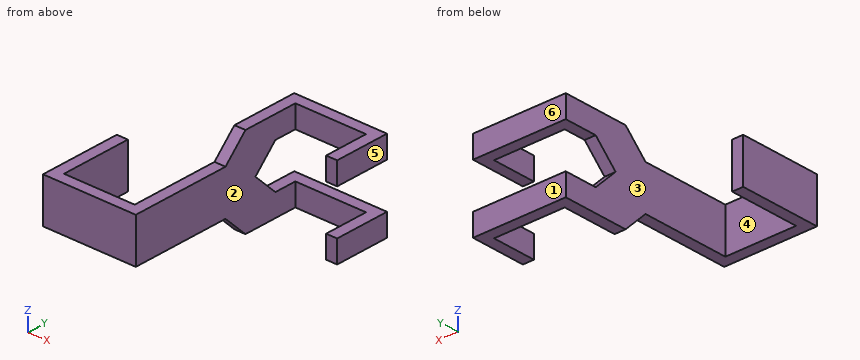
from build123d import *

# Parameters (mm, degrees)
F1_DEPTH = 5
F2_W     = 2.5
F2_H     = 2.5
F3_DEPTH = 5
F5_DEPTH = 2.5


with BuildPart() as f1:
    # F0 (on Top) → F1 (new body)
    with BuildSketch(Plane.XY):
        Polygon((-16, -30), (-16, 0), (-18.5, 0), (-18.5, -27.5), (-34.5, -27.5), (-34.5, -11.5), (-37, -11.5), (-37, -30), align=None)
    extrude(amount=F1_DEPTH)

    # F2 (on face) → F3 (join)
    with BuildSketch(Plane.XY.offset(5)):
        Polygon((2.5, 12.5), (-18.5, 12.5), (-18.5, 0), (-16, 0), (-16, 10), (0, 10), (0, 0), (2.5, 0), align=None)
        with Locations((-17.25, -1.25)):
            Rectangle(F2_W, F2_H)
    extrude(amount=F3_DEPTH)

    # F4 (on face) → F5 (join, through all)
    with BuildSketch(Plane(origin=(-18.5, 0, 0), x_dir=(0, -1, 0), z_dir=(-1, 0, 0))):
        Polygon((0, 5), (-5, 5), (0, 0), align=None)
        Polygon((7.5, 5), (2.5, 10), (2.5, 5), align=None)
    extrude(amount=-F5_DEPTH)

    # F6: F1 across plane


with BuildPart() as f1_1:
    add(f1.part)
    add(f1.part.mirror(Plane.XY))


solid = f1_1.part
Source: CAD feature listing. Evaluate the final solid. Frame: model axes, mm. Face numbers are marked on the shaded views. A direction names the side the tool comes from. Coordinates: 2 decimals unless noted, no trailing zeros. Loops run counter-clockwise (first coordinate to the right, second up) from the corner with the lowest first, then second, coordinate; pieces in that order, holes last. Notation, with made-up numbers: (75, 22.5) -> (122, 22.5) arc R15 ccw to (122, 33.5) -> close; hole circle Ø4 at (47, 76). An arc over 180 degrees is marked (long way). Answer in a Markdown table with one row per item. Add a question column.
Q1. Reachability of the marked faces 1, 2 and 3 from +Z, -Z, +X, -X, +Y, -Y: full face, straight path, thin tool, end or side. Return the list, or none.
Q2. Contact query for flat-ended pins moving along their axis: pin 1 Ø2.5 at (x, z) = (-10.5, 6.5) entering from -Y; pin 2 Ø3 at (x, z) = (2, -7) entering from -Y; pin 3 Ø5.5 at (y, z) = (5.5, -8) entering from -X. Output: stop coordinate, or through.
Q3. Section A-A on y = 0.5. Return the cut outline in (x, z).
Q4. Pull-direction query (X, two-part tool) for the marked faces 4, 5 and 6; classes: pulls with the +X half, pulls with the -X half, needs draft (parallel to the pull), parting line crosses it, or undercut.
Q5. Section D-D on y = -16. Return the cut outline in (x, z), and give its area (3 significant figures).
Q6. Section B-B on x = -2. Return the cut outline in (y, z).
Q7. Section C-C on z = 3.5. Return the cut outline in (x, y).
Q8. Ray query, line 1 along Z through (x, y) = (-14.5, 11); line 2 along X through (y, z) = (-22, 4.5); line 3 along X through (y, z) = (1.5, -8.25). Return the intervals inside material, ascending.
Computed values:
| question | item | result |
|---|---|---|
| 1 | face 1 | +Z, -Z, +X, -X, +Y |
| 1 | face 2 | +Z, -Z, -Y |
| 1 | face 3 | +Z, -Z, +Y |
| 2 | pin 1 | stops at y = 10 |
| 2 | pin 2 | stops at y = 0 |
| 2 | pin 3 | stops at x = -18.5 |
| 3 | outline | (-18.5, -10) -> (-16, -10) -> (-16, -0.5) -> (-18.5, -0.5) -> close; (-18.5, 0.5) -> (-16, 0.5) -> (-16, 10) -> (-18.5, 10) -> close; (0, -10) -> (2.5, -10) -> (2.5, -5) -> (0, -5) -> close; (0, 5) -> (2.5, 5) -> (2.5, 10) -> (0, 10) -> close |
| 4 | face 4 | undercut |
| 4 | face 5 | pulls with the +X half |
| 4 | face 6 | needs draft |
| 5 | outline | (-37, -5) -> (-34.5, -5) -> (-34.5, 5) -> (-37, 5) -> close; (-18.5, -5) -> (-16, -5) -> (-16, 5) -> (-18.5, 5) -> close |
| 5 | area | 50.0 mm^2 |
| 6 | outline | (10, -10) -> (12.5, -10) -> (12.5, -5) -> (10, -5) -> close; (10, 5) -> (12.5, 5) -> (12.5, 10) -> (10, 10) -> close |
| 7 | outline | (-37, -30) -> (-16, -30) -> (-16, 3.5) -> (-18.5, 3.5) -> (-18.5, -27.5) -> (-34.5, -27.5) -> (-34.5, -11.5) -> (-37, -11.5) -> close |
| 8 | line 1 | z = -10 to -5, 5 to 10 |
| 8 | line 2 | x = -37 to -34.5, -18.5 to -16 |
| 8 | line 3 | x = -18.5 to -16, 0 to 2.5 |
